from build123d import *

# Parameters (mm, degrees)
EXTRUDE_1_DEPTH     = 16
SKETCH_4_W          = 1.5
SKETCH_4_H          = 4.2
SKETCH_4_W_2        = 73.5
SKETCH_4_H_2        = 8.2
CUT_EXTRUDE_1_DEPTH = 10
FILLET_1_R          = 4.1
SKETCH_6_W          = 10
SKETCH_6_H          = 16
SKETCH_6_W_2        = 1.5
SKETCH_6_H_2        = 4.2
EXTRUDE_4_DEPTH     = 11
EXTRUDE_START       = -11
SKETCH_10_W         = 0.125
SKETCH_10_H         = 16
SKETCH_10_W_2       = 2.5
EXTRUDE_6_DEPTH     = 24
FILLET_2_R          = 3.5
FILLET_3_R          = 6


with BuildPart() as part:
    # 스케치1 → 보스-돌출1 (new body)
    with BuildSketch(Plane.XY):
        Polygon((-96, 0), (0, 0), (0, -21.5), (7.6, -21.5), (7.6, 5), (-96, 5), align=None)
    extrude(amount=EXTRUDE_1_DEPTH)

    # 스케치4 → 컷-돌출1 (cut)
    with BuildSketch(Plane.XZ):
        with Locations((-91, 8)):
            Rectangle(SKETCH_4_W, SKETCH_4_H)
        with Locations((-45.75, 8)):
            Rectangle(SKETCH_4_W_2, SKETCH_4_H_2)
    extrude(amount=-CUT_EXTRUDE_1_DEPTH, mode=Mode.SUBTRACT)

    # 필렛1
    fillet_1_edges = [part.edges().sort_by_distance(p)[0] for p in [
        (-82.5, 2.5, 3.9),
        (-82.5, 2.5, 12.1),
        (-9, 2.5, 3.9),
        (-9, 2.5, 12.1),
    ]]
    fillet(fillet_1_edges, radius=FILLET_1_R - 0.0001)  # a hair under: the kernel refuses the full size

    # 스케치6 → 보스-돌출4 (add)
    with BuildSketch(Plane(origin=(0, 5, 0), x_dir=(1, 0, 0), z_dir=(0, 1, 0))):
        with Locations((-91, -8)):
            Rectangle(SKETCH_6_W, SKETCH_6_H)
        with Locations((-91, -8)):
            Rectangle(SKETCH_6_W_2, SKETCH_6_H_2, mode=Mode.SUBTRACT)
    extrude(amount=-EXTRUDE_4_DEPTH)

    # 스케치10 → 보스-돌출6 (add)
    with BuildSketch(Plane.XZ.offset(6).offset(EXTRUDE_START)):
        with Locations((-95.9375, 8)):
            Rectangle(SKETCH_10_W, SKETCH_10_H)
        with Locations((-97.25, 8)):
            Rectangle(SKETCH_10_W_2, SKETCH_10_H)
        with Locations((-86.0625, 8)):
            Rectangle(SKETCH_10_W, SKETCH_10_H)
        with Locations((-84.75, 8)):
            Rectangle(SKETCH_10_W_2, SKETCH_10_H)
    extrude(amount=EXTRUDE_6_DEPTH)

    # 필렛2
    fillet_2_edges = [part.edges().sort_by_distance(p)[0] for p in [
        (-95.875, -6, 8),
        (-86.125, -6, 8),
    ]]
    fillet(fillet_2_edges, radius=FILLET_2_R)

    # 필렛3
    fillet_3_edges = [part.edges().sort_by_distance(p)[0] for p in [
        (0, 0, 8),
    ]]
    fillet(fillet_3_edges, radius=FILLET_3_R)


solid = part.part
The model under review builds one solid part; all positions refer to its coordinate system, in mm. A direction names the side the tool comes from. Round coordinates to 2 decimals unless told otherwise and drop trailing zeros. Loops run counter-clockwise (first coordinate to the right, second up) from the corner with the lowest first, then second, coordinate; pieces in that order, holes last. Notation, with made-up numbers: M -14,-38 L 41,-38 A10 ccw 41,-19 Z; hole C 16,-1 d2. An arc over 180 degrees is marked long. Answer as CSV lines item,"result".
1. Insertion check: pin 1 Ø0.8 at (x, z) = (-97.5, 6) entering from -Y; pin 2 Ø8 at (x, z) = (-55.5, 10.5) entering from -Y; pin 3 Ø3 at (x, z) = (-91, 4) entering from -Y. Each pin has a flat end and moves straight along its axis. Give the tip position at first contact, or say it passes through.
Outcome:
pin 1,"stops at y = -19"
pin 2,"stops at y = 0"
pin 3,"stops at y = -6"
2. We need section D-D (z = 1.5). Give the boundary of the cut face in (x, y) (3 decimals).
Outcome:
outline,"M -98.5,-19 L -95.875,-19 L -95.875,-9.5 A3.5 cw -92.375,-6 L -89.625,-6 A3.5 cw -86.125,-9.5 L -86.125,-19 L -83.5,-19 L -83.5,0 L -6,0 A6 cw 0,-6 L 0,-21.5 L 7.6,-21.5 L 7.6,5 L -98.5,5 Z"
3. To check wall thickness, follow L1, parallel to X at y = -10.5, z = 15.5 (3 decimals); L2, parallel to Y at x = -7, z = 9.75; L3, parallel to X at y = -7.5, z = 8.5. State the ranges of each line that lie inside material, in increasing order. Write a range as [from, to].
Outcome:
L1,"x = [-98.5, -95.875], [-86.125, -83.5], [0, 7.6]"
L2,"y = [0, 5]"
L3,"x = [-98.5, -95.25], [-86.75, -83.5], [0, 7.6]"
4. We need section A-A (y = -3.5). Give the boundary of the cut face in (x, z), plus the area to 3 significant figures.
Outcome:
outline,"M -98.5,0 L -83.5,0 L -83.5,16 L -98.5,16 Z; M -0.55,0 L 7.6,0 L 7.6,16 L -0.55,16 Z; hole M -91.75,5.9 L -90.25,5.9 L -90.25,10.1 L -91.75,10.1 Z"
area,"364 mm2"
5. We need section C-C (y = -16.25). Give the boundary of the cut face in (x, z) (3 decimals), plus the area to 3 significant figures.
Outcome:
outline,"M -98.5,0 L -95.875,0 L -95.875,16 L -98.5,16 Z; M -86.125,0 L -83.5,0 L -83.5,16 L -86.125,16 Z; M 0,0 L 7.6,0 L 7.6,16 L 0,16 Z"
area,"206 mm2"
6. We need section B-B (x = -32). Give the boundary of the cut face in (y, z), plus the area to 3 significant figures.
Outcome:
outline,"M 0,0 L 5,0 L 5,3.9 L 0,3.9 Z; M 0,12.1 L 5,12.1 L 5,16 L 0,16 Z"
area,"39.0 mm2"
7. For faces 5 (the face through (-90.25, -1, 8)), 6 (the face through (7.6, -8, 8)), 7 (the face through (-1.711, -1.804, 8.112)), 8 (the face through (-97, -19, 8)), list the 3-axis set-ups (+Z, -Z, +X, -X, +Y, -Y) from which the entire face can be reached by the end or side of a thin tool; tool diameter is ignored.
Outcome:
face 5,"+Y, -Y"
face 6,"+Z, -Z, +X, +Y, -Y"
face 7,"+Z, -Z, -Y"
face 8,"+Z, -Z, -X, -Y"
8. Draft analysis for pull direction Z (two halves, no side actions). For faces 1 (the face through (-81.3, 2.5, 5.1)), 2 (the face through (-45, 5, 13)), 3 (the face through (-46, 3, 0)), 4 (the face through (-46, 3, 16)), state which applies: pulls with the +Z half, pulls with the -Z half, needs draft (parallel to the pull), parting line crosses it, or undercut.
Outcome:
face 1,"undercut"
face 2,"needs draft"
face 3,"pulls with the -Z half"
face 4,"pulls with the +Z half"
